The model under review builds one solid part; all positions refer to its coordinate system, in mm. A direction names the side the tool comes from. Round coordinates to 2 decimals unless told otherwise and drop trailing zeros. Order: outer loops, then holes, each group sorted by start corner. A loop starts at its lowest first (then second) coordinate and runs counter-clockwise, first axis right, second up. Notation, with made-up numbers: M 38.25,70.25 L 85.25,70.25 A10 cw 85.25,88.25 Z; hole C 22,33 d7. An arc over 180 degrees is marked long. Use a Markdown table: item, result. Add a question column.
1. To check wall thickness, follow probe 1 along X at (y, z) = (0, -6.5); probe 2 along Y at (x, z) = (0, -5); probe 3 along Y at (x, z) = (-0.1, -15). State the ranges of each line that lie inside material, in increasing order.
2. For faces 4 (the cylindrical face through (-0.02, -1.86, -14.35)), 5 (the cylindrical face through (0, 3, 1)), 6 (the flat face through (-1.5, 1, -16)), 7 (the cylindrical face through (0, 1.1, -5.9)), list the 3-axis set-ups (+Z, -Z, +X, -X, +Y, -Y) from which the entire face can be reached by the end or side of a thin tool; tool diameter is ignored.
3. Consider section C-C on z = -15.75. State the section outline as (x, y) points.
4. Insertion check: P1, Ø3, axis at y = 0, z = -15, coming from the -X side; P2, Ø1.8, axis at x = 0, y = 0, coming from the +Z side; P3, Ø1.5, axis at x = -1, z = -6.5, coming from the -Y side. Each pin has a flat end and moves straight along its axis. Give the tip position at first contact, or say it passes through.
5. Consider section A-A on z = 0. State the section outline as (x, y) points, then the cut area to 3 significant figures.
6. Consider section D-D on y = 1.75. State the section outline as (x, z) points.
7. The part is to be moulded in two halves that separate along Z. For faces 1 (the cylindrical face through (-0.03, -1.56, -13.06)), 2 (the flat face through (0, -1.4, 3)), 3 (the flat face through (1.5, 1, -16)), say which applies: +Z half, -Z half, draft (parallel to the pull), parting line (faces both ways), or undercut.
8. Consider section B-B on x = 0.75. State the section outline as (y, z) points.
Autodesk Inventor part; units mm, degrees
ref_plane "YZ Plane" through (0, 0, 0) normal (1, 0, 0) x (0, 1, 0)
ref_plane "XZ Plane" through (0, 0, 0) normal (0, 1, 0) x (-1, 0, 0)
ref_plane "XY Plane" through (0, 0, 0) normal (0, 0, 1) x (1, 0, 0)
sketch "スケッチ1" plane through (0, 0, 0) normal (0, 1, 0) x (-1, 0, 0)
  line L0 (2.5, 3) -> (-2.5, 3)
  line L1 (-2.5, 3) -> (-2.5, -12)
  line L2 (-2.5, -12) -> (2.5, -12)
  line L3 (2.5, -12) -> (2.5, 3)
  point P0 (0, 0)
  point P1 (0, 3)
  dimension "d0" = 5
  dimension "d15" = 15
  dimension "d46" = 3
extrude "押し出し1" add sketch "スケッチ1" along normal mid plane 4
sketch "スケッチ2" plane through (0, 0, 0) normal (0, 1, 0) x (-1, 0, 0)
  circle A0 centre (0, 0) radius 1
  dimension "d3" = 2
extrude "押し出し2" add sketch "スケッチ2" along normal mid plane 6.5
sketch "スケッチ5" plane through (-2.5, 2, 3) normal (0, 0, 1) x (1, 0, 0)
  point P0 (2.5, -2)
  point P1 (2.5, -2)
hole "加工用" [suppressed]
sketch "スケッチ8" plane through (0, 0, 0) normal (1, 0, 0) x (0, 1, 0)
  circle A0 centre (0, -15) radius 2.5
  circle A1 centre (0, -15) radius 1.2
  line L0 (-2, -12) -> (-2.4604, -14.557)
  line L1 (2, -12) -> (2.4604, -14.557)
  line L2 (-2, -12) -> (2, -12)
  line L3 (-2, -12) -> (2, -12)
  circle A2 centre (-1.85, -15) radius 0.65
  arc A3 (-2, -12) -> (0, -13.8) centre (0, -11.7889) ccw
  point P0 (0, 0)
  point P1 (1, -4)
  point P2 (-1, -4)
  point P3 (0, -12)
  point P4 (0, -12)
  point P5 (-1.2, -15)
  point P6 (-2.5, -15)
  point P7 (0, -12)
  point P8 (-1.5657, -13.051)
  dimension "d33" = 2.4
  dimension "d34" = 5
  dimension "d42" = 3
extrude "押し出し4" add sketch "スケッチ8" along normal mid plane 3 contours A0 A2 A1 A3 | A0 A3 L2 L1 | A2 picked at (-1.463, -16.0204)
fillet "フィレット1" radius 2 4 edges at (-1.5, 0, -12) (-2.5, 0, -12) (1.5, 0, -12) (2.5, 0, -12)
sketch "スケッチ6" plane through (-2.5, 2, 3) normal (0, 0, 1) x (1, 0, 0)
  point P0 (2.5, -2)
  point P1 (2.5, -2)
hole "穴3" at (0, 0, 3) direction (0, 0, -1) diameter 2.2 end up to surface
properties part number "gear_2" material "ABS プラスチック"
Answer block:
| question | item | result |
|---|---|---|
| 1 | probe 1 | -2.5 to -1.1, 1.1 to 2.5 |
| 1 | probe 2 | -2 to -1.1, 1.1 to 2 |
| 1 | probe 3 | -2.5 to -1.2, 1.2 to 2.5 |
| 2 | face 4 | +X, -X |
| 2 | face 5 | +Y |
| 2 | face 6 | -Z, -X, +Y, -Y |
| 2 | face 7 | +Z |
| 3 | outline | M -1.5,-2.38 L 1.5,-2.38 L 1.5,-0.94 L -1.5,-0.94 Z; M -1.5,0.94 L 1.5,0.94 L 1.5,2.38 L -1.5,2.38 Z |
| 4 | P1 | x = -1.51 |
| 4 | P2 | z = -15.79 |
| 4 | P3 | y = -2 |
| 5 | outline | M -2.5,-2 L -1,-2 L -1,-3.25 L 1,-3.25 L 1,-2 L 2.5,-2 L 2.5,2 L 1,2 L 1,3.25 L -1,3.25 L -1,2 L -2.5,2 Z; hole C 0,0 d2.2 |
| 5 | area | 21.2 mm^2 |
| 6 | outline | M -2.5,-11.09 A2 ccw -2,-12.41 A2 cw -1.5,-13.73 L -1.5,-16.79 L 1.5,-16.79 L 1.5,-13.73 A2 cw 2,-12.41 A2 ccw 2.5,-11.09 L 2.5,3 L -2.5,3 Z |
| 7 | face 1 | undercut |
| 7 | face 2 | +Z half |
| 7 | face 3 | draft |
| 8 | outline | M -3.25,-0.66 L -2,-0.66 L -2,-12 A2.01 ccw -0.8,-13.63 L -0.8,3 L -2,3 L -2,0.66 L -3.25,0.66 Z; M -2.5,-15 A2.5 ccw long 2.46,-14.56 L 2,-12 L 2,-0.66 L 3.25,-0.66 L 3.25,0.66 L 2,0.66 L 2,3 L 0.8,3 L 0.8,-14.11 A1.2 cw long -1.2,-15 A0.65 ccw Z |
